from build123d import *


with BuildPart() as part:
    # Szkic1 → Obrót1 (revolve)
    with BuildSketch(Plane.XY):
        with BuildLine():
            Line((-12, 12), (-9.3, 12))
            Line((-9.3, 12), (-9.3, 12.6))
            Line((-9.3, 12.6), (-8, 12.6))
            Line((-8, 12.6), (-8, 12))
            Line((-8, 12), (8, 12))
            Line((8, 12), (8, 10.5))
            Line((8, 10.5), (10, 10.5))
            Line((10, 10.5), (10, 12))
            Line((10, 12), (12, 12))
            Line((12, 12), (12, 13.35))
            Line((12, 13.35), (8.5, 13.35))
            Line((8.5, 13.35), (8.5, 16.5))
            Line((8.5, 16.5), (7.5, 16.5))
            Line((7.5, 16.5), (7.5, 16))
            ThreePointArc((7.5, 16), (6.914213562, 14.585786438), (5.5, 14))
            Line((5.5, 14), (-5.5, 14))
            ThreePointArc((-5.5, 14), (-6.914213562, 14.585786438), (-7.5, 16))
            Line((-7.5, 16), (-7.5, 16.5))
            Line((-7.5, 16.5), (-8.5, 16.5))
            Line((-8.5, 16.5), (-8.5, 13.35))
            Line((-8.5, 13.35), (-12, 13.35))
            Line((-12, 13.35), (-12, 12))
        make_face()
    revolve(axis=Axis((-7.001985985, 0, 0), (1, 0, 0)))


solid = part.part
Geometry: final body of the model. Coordinates: model frame, mm. A direction names the side the tool comes from. Round coordinates to 2 decimals unless told otherwise and drop trailing zeros. Loops run counter-clockwise (first coordinate to the right, second up) from the corner with the lowest first, then second, coordinate; pieces in that order, holes last.
Q1. Material intervals for L1, parallel to Z at x = -11.3, y = 0; L2, parallel to X at y = -13, z = -10; L3, parallel to Z at x = -8.7, y = 0, sorted ascending.
Q2. Section A-A on x = 0.5. Return loops of the section in (y, z).
Q3. Pin query (flat end, axial travel): P1, Ø2, axis at x = -7, y = -2, coming from the +Z side; P2, Ø8, axis at x = -2, y = -12.5, coming from the +Z side; P3, Ø16.5, axis at y = 3.5, z = 0, coming from the -X side. Return the tip coordinate at first contact, or that it passes through.
Q4. Access query for faces 1 (the cylindrical face through (11.01, -11.99, 0.53)), 2 (the cylindrical face through (-8.641, -9.999, -7.667)), 3 (the flat face through (12, 12, 2)), 4 (the cylindrical face through (-10.274, 12.734, 4.01)), 5 (the flat face through (-12, -12, 2)). Directions: +Z, -Z, +X, -X, +Y, -Y. A direction counts if a zero-diameter tool reaches every point of the face in a straight line with its end or side. Return the directions, or none.
Q5. Pull-direction query (X, two-part tool) for faces 6 (the flat face through (7.5, -16, 3)), 7 (the flat face through (-7.5, 16, 3)), 8 (the flat face through (8.5, -6, -12.1)), 9 (the cylindrical face through (10.226, 12.734, 4.01)); classes: released by +X, released by -X, zero draft, split by the parting line, or undercut.
Evaluation:
1. L1: z = -13.35 to -12, 12 to 13.35
1. L2: x = -8.5 to -7.5, 7.5 to 8.5
1. L3: z = -13.35 to -12.6, 12.6 to 13.35
2. outline: circle Ø28 at (0, 0); hole circle Ø24 at (0, 0)
3. P1: stops at z = 16.46
3. P2: stops at z = 11.12
3. P3: stops at x = 8
4. face 1: +X
4. face 2: none
4. face 3: +Z, -Z, +X, +Y, -Y
4. face 4: -X
4. face 5: +Z, -Z, -X, +Y, -Y
5. face 6: undercut
5. face 7: undercut
5. face 8: released by +X
5. face 9: zero draft
